```python
from build123d import *

# Parameters (mm, degrees)
SKETCH1_R           = 2.413
BOSS_EXTRUDE1_DEPTH = 6.35
BOSS_EXTRUDE2_START = 4.762246
SKETCH2_R           = 2.413
BOSS_EXTRUDE2_DEPTH = 4.762246
SKETCH3_R           = 3.175
BOSS_EXTRUDE3_DEPTH = 3.175
SKETCH4_R           = 3.175
BOSS_EXTRUDE4_DEPTH = 3.175
THREAD2_PITCH       = 1.27
SKETCH11_R          = 6.35
BOSS_EXTRUDE5_DEPTH = 3.81
CUT_EXTRUDE1_START  = -0.952246
SKETCH13_R          = 2.413
CUT_EXTRUDE1_DEPTH  = 0.952246
SKETCH14_R          = 2.413
BOSS_EXTRUDE6_DEPTH = 2.54
SKETCH16_W          = 13.786641265
SKETCH16_H          = 13.864798174
SKETCH16_W_2        = 7.9375
SKETCH16_H_2        = 7.9375
CUT_EXTRUDE3_DEPTH  = 3.81
CUT_EXTRUDE4_START  = -6.35
SKETCH17_R          = 2.413
SKETCH17_R_2        = 2.159
CUT_EXTRUDE4_DEPTH  = 6.35


with BuildPart() as part:
    # Sketch1 → Boss-Extrude1 (new body)
    with BuildSketch(Plane(origin=(0, 0, 0), x_dir=(1, 0, 0), z_dir=(0, 1, 0))):
        with Locations(Location((0, 0, 0), (0, 0, 270))):
            Circle(SKETCH1_R)
    extrude(amount=BOSS_EXTRUDE1_DEPTH)

    # Sketch2 → Boss-Extrude2 (add)
    with BuildSketch(Plane(origin=(0, 0, 0), x_dir=(-1, 0, 0), z_dir=(0, -1, 0)).offset(BOSS_EXTRUDE2_START)):
        with Locations(Location((0, 0, 0), (0, 0, 90))):
            Circle(SKETCH2_R)
    extrude(amount=-BOSS_EXTRUDE2_DEPTH)

    # Sketch3 → Boss-Extrude3 (add)
    with BuildSketch(Plane(origin=(0, -4.762246, 0), x_dir=(-1, 0, 0), z_dir=(0, -1, 0))):
        with Locations(Location((0, 0, 0), (0, 0, 90))):
            Circle(SKETCH3_R)
    extrude(amount=BOSS_EXTRUDE3_DEPTH)

    # Sketch4 → Boss-Extrude4 (add)
    with BuildSketch(Plane(origin=(0, -7.937246, 0), x_dir=(-1, 0, 0), z_dir=(0, -1, 0))):
        with Locations(Location((0, 0, 0), (0, 0, 90))):
            Circle(SKETCH4_R)
    extrude(amount=BOSS_EXTRUDE4_DEPTH)

    # Thread2: the profile of Thread Profile3 profile screwed along a right-hand helix of 3.75 turns, 8 arcs to a turn; built about Z, then put on its axis
    thread2_z = Axis((0, 0, 0), (0, 0, 1))
    thread2_corners = [(3.1753, 0, -0.000173205), (3.1753, 0, 1.111423202), (2.487592339, 0, 0.714374998), (2.487592339, 0, 0.396874998)]
    with BuildLine(mode=Mode.PRIVATE) as thread2_profile:
        Line(thread2_corners[0], thread2_corners[1])
        Line(thread2_corners[1], thread2_corners[2])
        Line(thread2_corners[2], thread2_corners[3])
        Line(thread2_corners[3], thread2_corners[0])
    thread2_cap = Face(thread2_profile.wire())
    thread2_turn_angles = [0, 22.5, 45, 67.5, 90, 112.5, 135, 157.5, 180, 202.5, 225, 247.5, 270, 292.5, 315, 337.5, 360]
    thread2_turn_weights = [1, 0.9238795325112867, 1, 0.9238795325112867, 1, 0.9238795325112867, 1, 0.9238795325112867, 1, 0.9238795325112867, 1, 0.9238795325112867, 1, 0.9238795325112867, 1, 0.9238795325112867, 1]
    thread2_turn_rails = [Edge.make_bspline([Vector(p[0], p[1], 0).rotate(thread2_z, thread2_turn_angles[k]) / thread2_turn_weights[k] + Vector(0, 0, p[2] + THREAD2_PITCH * thread2_turn_angles[k] / 360) for k in range(17)], [0, 0, 0, 1, 1, 2, 2, 3, 3, 4, 4, 5, 5, 6, 6, 7, 7, 8, 8, 8], 2, thread2_turn_weights) for p in thread2_corners]
    thread2_turn_sides = [Face.make_surface_from_curves(thread2_turn_rails[p[0]], thread2_turn_rails[p[1]]) for p in [(0, 1), (1, 2), (2, 3), (3, 0)]]
    thread2_last_angles = [1080, 1102.5, 1125, 1147.5, 1170, 1192.5, 1215, 1237.5, 1260, 1282.5, 1305, 1327.5, 1350]
    thread2_last_weights = [1, 0.9238795325112867, 1, 0.9238795325112867, 1, 0.9238795325112867, 1, 0.9238795325112867, 1, 0.9238795325112867, 1, 0.9238795325112883, 1]
    thread2_last_rails = [Edge.make_bspline([Vector(p[0], p[1], 0).rotate(thread2_z, thread2_last_angles[k]) / thread2_last_weights[k] + Vector(0, 0, p[2] + THREAD2_PITCH * thread2_last_angles[k] / 360) for k in range(13)], [0, 0, 0, 1, 1, 2, 2, 3, 3, 4, 4, 5, 5, 6, 6, 6], 2, thread2_last_weights) for p in thread2_corners]
    thread2_last_sides = [Face.make_surface_from_curves(thread2_last_rails[p[0]], thread2_last_rails[p[1]]) for p in [(0, 1), (1, 2), (2, 3), (3, 0)]]
    thread2 = Plane(origin=(0, -9.524746, 0), x_dir=(1, 0, 0), z_dir=(0, 1, 0)) * Solid(Shell([*[p.moved(Location((0, 0, THREAD2_PITCH * i))) for i in range(3) for p in thread2_turn_sides], *thread2_last_sides, thread2_cap, thread2_cap.rotate(thread2_z, 1350).moved(Location((0, 0, THREAD2_PITCH * 1350 / 360)))]))
    add(thread2, mode=Mode.SUBTRACT)

    # Sketch11 → Boss-Extrude5 (add)
    with BuildSketch(Plane(origin=(0, -11.112246, 0), x_dir=(-1, 0, 0), z_dir=(0, -1, 0))):
        with Locations(Location((0, 0, 0), (0, 0, 270))):
            Circle(SKETCH11_R)
    extrude(amount=BOSS_EXTRUDE5_DEPTH)

    # Sketch13 → Cut-Extrude1 (cut)
    with BuildSketch(Plane(origin=(0, 6.35, 0), x_dir=(1, 0, 0), z_dir=(0, 1, 0)).offset(CUT_EXTRUDE1_START)):
        with Locations(Location((0, 0, 0), (0, 0, 90))):
            Circle(SKETCH13_R)
    extrude(amount=CUT_EXTRUDE1_DEPTH, mode=Mode.SUBTRACT)

    # Sketch14 → Boss-Extrude6 (add)
    with BuildSketch(Plane(origin=(0, 5.397754, 0), x_dir=(1, 0, 0), z_dir=(0, 1, 0))):
        with Locations(Location((0, 0, 0), (0, 0, 90))):
            Circle(SKETCH14_R)
    extrude(amount=BOSS_EXTRUDE6_DEPTH)

    # Sketch16 → Cut-Extrude3 (cut)
    with BuildSketch(Plane.XZ.offset(14.922246)):
        with Locations((-0.248819293, 0.124312734)):
            Rectangle(SKETCH16_W, SKETCH16_H)
        Rectangle(SKETCH16_W_2, SKETCH16_H_2, mode=Mode.SUBTRACT)
    extrude(amount=-CUT_EXTRUDE3_DEPTH, mode=Mode.SUBTRACT)

    # Sketch17 → Cut-Extrude4 (cut)
    with BuildSketch(Plane(origin=(0, 7.937754, 0), x_dir=(1, 0, 0), z_dir=(0, 1, 0)).offset(CUT_EXTRUDE4_START)):
        with Locations(Location((0, 0, 0), (0, 0, 90))):
            Circle(SKETCH17_R)
        with Locations(Location((0, 0, 0), (0, 0, 270))):
            Circle(SKETCH17_R_2, mode=Mode.SUBTRACT)
    extrude(amount=CUT_EXTRUDE4_DEPTH, mode=Mode.SUBTRACT)


solid = part.part
```
The model under review builds one solid part; all positions refer to its coordinate system, in mm. A direction names the side the tool comes from. Round coordinates to 2 decimals unless told otherwise and drop trailing zeros. Write each loop counter-clockwise with the first axis right and the second up, starting at its lowest first coordinate (ties: lowest second). Pieces come first, ordered by that corner, then holes. Notation, with made-up numbers: (-26, 21.25) - (-10, 21.25) arc R19 cw to (-10, 49.25) - close; hole circle Ø2 at (46.5, 81.25). An arc over 180 degrees is marked (long way). Answer as CSV lines item,"result". Start each with the question number.
(1) For faces 1 (the cylindrical face through (2.14, 4.72, -0.28)), 2 (the flat face through (0, 7.938, 0)), list the 3-axis set-ups (+Z, -Z, +X, -X, +Y, -Y) from which the entire face can be reached by the end or side of a thin tool; tool diameter is ignored.
(2) For pin 1 Ø1.5 at (x, y) = (-3, 3.5) entering from -Z; pin 2 Ø4 at (x, y) = (-1, 3) entering from -Z; pin 3 Ø4 at (y, z) = (-2.5, -3) entering from -X, all flat-tipped, find the tip position at first contact; note any pin that passes through.
(3) We need section A-A on z = 2.75. Give the number of separate pieces and of enclosed holes in the cut face, plus the area to 3 significant figures.
(4) We need section B-B on y = 1.25. State the section outline as (x, z) points, plus the area to 3 significant figures.
(5) To check wall thickness, follow line 1 (Y direction, x = 3, z = 0.25); line 2 (Y direction, x = -2, z = 2); line 3 (Y direction, x = 3.25, z = 2.5). State the ranges of each line that lie inside material, in increasing order.
Worked answers:
1,face 1,"+Y"
1,face 2,"+Z, -Z, +X, -X, +Y"
2,pin 1,"through"
2,pin 2,"z = -2.41"
2,pin 3,"x = -2.2"
3,separate pieces,"4"
3,enclosed holes,"0"
3,area,"42.9 mm²"
4,outline,"circle Ø4.83 at (0, 0)"
4,area,"18.3 mm²"
5,line 1,"-14.92 to -8.18, -7.25 to -6.91, -5.98 to -5.64"
5,line 2,"-14.92 to -8.53, -7.82 to -7.26, -6.55 to -5.99, -5.28 to -4.76"
5,line 3,"-14.92 to -11.11"
